Geometry check sheet. Reference: the model listing, model coordinates, mm. A direction names the side the tool comes from. Round coordinates to 2 decimals unless told otherwise and drop trailing zeros. Write each loop counter-clockwise with the first axis right and the second up, starting at its lowest first coordinate (ties: lowest second). Pieces come first, ordered by that corner, then holes. Notation, with made-up numbers: M 4,62.25 L 19,62.25 A19 cw 19,74.25 Z; hole C -7.5,22 d2. An arc over 180 degrees is marked long. Answer as CSV lines item,"result". Start each with the question number.
```python
from build123d import *

# Parameters (mm, degrees)
SKETCH1_W                  = 40
SKETCH1_H                  = 22
BOSS_EXTRUDE1_DEPTH        = 11
SKETCH2_W                  = 40
SKETCH2_H                  = 22
SKETCH2_R                  = 4
BOSS_EXTRUDE2_DEPTH        = 5
SKETCH3_W                  = 24.5
SKETCH3_H                  = 15.5
CUT_EXTRUDE1_DEPTH         = 7.75
FILLET1_R                  = 7.75
SKETCH4_R                  = 5
CUT_EXTRUDE2_DEPTH         = 36.805900352
SKETCH5_W                  = 8
SKETCH5_H                  = 8
SKETCH5_R                  = 1.905800151
BOSS_EXTRUDE3_DEPTH        = 6
CUT_EXTRUDE3_START         = -3
SKETCH6_R                  = 3
SKETCH6_R_2                = 1.905800151
CUT_EXTRUDE3_DEPTH         = 3
SKETCH7_W                  = 16
SKETCH7_H                  = 16.5
BOSS_EXTRUDE5_DEPTH        = 28
MIRROR14_COPY_1_SKETCH_W   = 8
MIRROR14_COPY_1_SKETCH_H   = 8
MIRROR14_COPY_1_SKETCH_R   = 1.905800151
MIRROR14_COPY_1_DEPTH      = 6
MIRROR14_START             = -3
MIRROR14_COPY_2_SKETCH_R   = 3
MIRROR14_COPY_2_SKETCH_R_2 = 1.905800151
MIRROR14_COPY_2_DEPTH      = 3
FILLET1_OF_MIRROR14_R      = 7.75
SKETCH9_W                  = 28
SKETCH9_H                  = 3
BOSS_EXTRUDE6_DEPTH        = 18
CUT_EXTRUDE4_DEPTH         = 10
CUT_EXTRUDE5_DEPTH         = 73.919476136
CUT_EXTRUDE5_DEPTH_BACK    = 73.919476136
SKETCH11_R                 = 1.75
CUT_EXTRUDE6_DEPTH         = 76.121568141
CUT_EXTRUDE6_DEPTH_BACK    = 76.121568141
SKETCH12_R                 = 1.75
FILLET2_R                  = 2
CUT_EXTRUDE12_START        = -3
SKETCH17_R                 = 1.75
CUT_EXTRUDE12_DEPTH        = 3
CUT_EXTRUDE13_DEPTH        = 74.097537578
CUT_EXTRUDE13_DEPTH_BACK   = 74.097537578
SKETCH18_W                 = 18
SKETCH18_H                 = 5
FILLET3_R                  = 2.5
CUT_EXTRUDE14_DEPTH        = 74.710582687
CUT_EXTRUDE15_START        = -10
SKETCH21_R                 = 1.75
CUT_EXTRUDE15_DEPTH        = 10
SKETCH20_W                 = 36.163748027
SKETCH20_H                 = 4
CUT_EXTRUDE16_DEPTH        = 13.5
SKETCH22_W                 = 6.75
SKETCH22_H                 = 13.5
CUT_EXTRUDE18_DEPTH        = 8


with BuildPart() as part:
    # Sketch1 → Boss-Extrude1 (new body)
    with BuildSketch(Plane(origin=(0, 0, 0), x_dir=(1, 0, 0), z_dir=(0, 1, 0))):
        Rectangle(SKETCH1_W, SKETCH1_H)
    boss_extrude1 = extrude(amount=BOSS_EXTRUDE1_DEPTH)

    # Sketch2 → Boss-Extrude2 (add)
    with BuildSketch(Plane(origin=(0, 0, 0), x_dir=(1, 0, 0), z_dir=(0, 1, 0))):
        Rectangle(SKETCH2_W, SKETCH2_H)
        with Locations(Location((0, 0, 0), (0, 0, 270))):
            Circle(SKETCH2_R, mode=Mode.SUBTRACT)
    boss_extrude2 = extrude(amount=-BOSS_EXTRUDE2_DEPTH)

    # Sketch3 → Cut-Extrude1 (cut)
    with BuildSketch(Plane(origin=(0, 11, 0), x_dir=(1, 0, 0), z_dir=(0, 1, 0))):
        Rectangle(SKETCH3_W, SKETCH3_H)
    cut_extrude1 = extrude(amount=-CUT_EXTRUDE1_DEPTH, mode=Mode.SUBTRACT)

    # Fillet1
    fillet1_edges = [part.edges().sort_by_distance(p)[0] for p in [
        (0, 3.25, 7.75),
        (0, 3.25, -7.75),
    ]]
    fillet(fillet1_edges, radius=FILLET1_R - 0.0001)  # a hair under: the kernel refuses the full size

    # Sketch4 → Cut-Extrude2 (cut, symmetric)
    with BuildSketch(Plane(origin=(-12.25, 0, 0), x_dir=(0, 0, -1), z_dir=(1, 0, 0))):
        with Locations((0, 11)):
            Circle(SKETCH4_R)
    cut_extrude2 = extrude(amount=CUT_EXTRUDE2_DEPTH, both=True, mode=Mode.SUBTRACT)

    # Sketch5 → Boss-Extrude3 (add)
    with BuildSketch(Plane(origin=(0, 11, 0), x_dir=(1, 0, 0), z_dir=(0, 1, 0))):
        with Locations((16, -15)):
            Rectangle(SKETCH5_W, SKETCH5_H)
        with Locations(Location((16, -15, 0), (0, 0, 270))):
            Circle(SKETCH5_R, mode=Mode.SUBTRACT)
    boss_extrude3 = extrude(amount=-BOSS_EXTRUDE3_DEPTH)

    # Sketch6 → Cut-Extrude3 (cut)
    with BuildSketch(Plane.XZ.offset(-5).offset(CUT_EXTRUDE3_START)):
        with Locations(Location((16, 15, 0), (0, 0, 270))):
            Circle(SKETCH6_R)
        with Locations(Location((16, 15, 0), (0, 0, 90))):
            Circle(SKETCH6_R_2, mode=Mode.SUBTRACT)
    cut_extrude3 = extrude(amount=CUT_EXTRUDE3_DEPTH, mode=Mode.SUBTRACT)

    # Mirror8: Boss-Extrude3, Cut-Extrude3 across plane
    add(boss_extrude3.mirror(Plane(origin=(0, 0, 0), x_dir=(0, 0, 1), z_dir=(1, 0, 0))))
    add(cut_extrude3.mirror(Plane(origin=(0, 0, 0), x_dir=(0, 0, 1), z_dir=(1, 0, 0))), mode=Mode.SUBTRACT)

    # Sketch7 → Boss-Extrude5 (add)
    with BuildSketch(Plane(origin=(0, 0, -11), x_dir=(-1, 0, 0), z_dir=(0, 0, -1))):
        with Locations((-12, 9.25)):
            Rectangle(SKETCH7_W, SKETCH7_H)
    extrude(amount=BOSS_EXTRUDE5_DEPTH)

    # Mirror14: Boss-Extrude1, Boss-Extrude2, Cut-Extrude1, Cut-Extrude2, Boss-Extrude3, Cut-Extrude3 across plane
    add(boss_extrude1.mirror(Plane.XY.offset(-25)))
    add(boss_extrude2.mirror(Plane.XY.offset(-25)))
    add(cut_extrude1.mirror(Plane.XY.offset(-25)), mode=Mode.SUBTRACT)
    add(cut_extrude2.mirror(Plane.XY.offset(-25)), mode=Mode.SUBTRACT)
    add(boss_extrude3.mirror(Plane.XY.offset(-25)))
    add(cut_extrude3.mirror(Plane.XY.offset(-25)), mode=Mode.SUBTRACT)

    # Mirror14 copy 1 sketch → Mirror14 copy 1 (add)
    with BuildSketch(Plane(origin=(0, 11, -50), x_dir=(-1, 0, 0), z_dir=(0, 1, 0))):
        with Locations((16, -15)):
            Rectangle(MIRROR14_COPY_1_SKETCH_W, MIRROR14_COPY_1_SKETCH_H)
        with Locations(Location((16, -15, 0), (0, 0, 270))):
            Circle(MIRROR14_COPY_1_SKETCH_R, mode=Mode.SUBTRACT)
    extrude(amount=-MIRROR14_COPY_1_DEPTH)

    # Mirror14 copy 2 sketch → Mirror14 copy 2 (cut)
    with BuildSketch(Plane(origin=(0, 5, -50), x_dir=(-1, 0, 0), z_dir=(0, -1, 0)).offset(MIRROR14_START)):
        with Locations(Location((16, 15, 0), (0, 0, 270))):
            Circle(MIRROR14_COPY_2_SKETCH_R)
        with Locations(Location((16, 15, 0), (0, 0, 90))):
            Circle(MIRROR14_COPY_2_SKETCH_R_2, mode=Mode.SUBTRACT)
    extrude(amount=MIRROR14_COPY_2_DEPTH, mode=Mode.SUBTRACT)

    # Fillet1 of Mirror14
    fillet1_of_mirror14_edges = [part.edges().sort_by_distance(p)[0] for p in [
        (0, 3.25, -57.75),
        (0, 3.25, -42.25),
    ]]
    fillet(fillet1_of_mirror14_edges, radius=FILLET1_OF_MIRROR14_R - 0.0001)  # a hair under: the kernel refuses the full size

    # Sketch9 → Boss-Extrude6 (add)
    with BuildSketch(Plane.ZY.offset(-4)):
        with Locations((-25, 2.5)):
            Rectangle(SKETCH9_W, SKETCH9_H)
    extrude(amount=BOSS_EXTRUDE6_DEPTH)

    # Sketch10 → Cut-Extrude4 (cut)
    with BuildSketch(Plane(origin=(0, 17.5, 0), x_dir=(1, 0, 0), z_dir=(0, 1, 0))):
        with BuildLine():
            Line((9, 26.25), (9, 23.75))
            Line((9, 23.75), (11.727178029, 23.75))
            ThreePointArc((11.727178029, 23.75), (11.931001031, 24.360286817), (12, 25))
            ThreePointArc((12, 25), (11.931001031, 25.639713183), (11.727178029, 26.25))
            Line((11.727178029, 26.25), (9, 26.25))
        make_face()
        with BuildLine():
            Line((11.727178029, 23.75), (9, 23.75))
            Line((9, 23.75), (9, 26.25))
            Line((9, 26.25), (11.727178029, 26.25))
            ThreePointArc((11.727178029, 26.25), (6, 25), (11.727178029, 23.75))
        make_face()
        with BuildLine():
            ThreePointArc((12, 25), (11.931001031, 24.360286817), (11.727178029, 23.75))
            Line((11.727178029, 23.75), (20, 23.75))
            Line((20, 23.75), (20, 26.25))
            Line((20, 26.25), (11.727178029, 26.25))
            ThreePointArc((11.727178029, 26.25), (11.931001031, 25.639713183), (12, 25))
        make_face()
    extrude(amount=-CUT_EXTRUDE4_DEPTH, mode=Mode.SUBTRACT)

    # Sketch11 → Cut-Extrude5 (cut, two sides: drawn at the far end of the back side and taken through both)
    with BuildSketch(Plane(origin=(0, 7.5, 0), x_dir=(1, 0, 0), z_dir=(0, 1, 0)).offset(-CUT_EXTRUDE5_DEPTH_BACK)):
        with Locations(Location((9, 25, 0), (0, 0, 270))):
            Circle(SKETCH11_R)
    extrude(amount=CUT_EXTRUDE5_DEPTH + CUT_EXTRUDE5_DEPTH_BACK, mode=Mode.SUBTRACT)

    # Sketch12 → Cut-Extrude6 (cut, two sides: drawn at the far end of the back side and taken through both)
    with BuildSketch(Plane.ZY.offset(-4).offset(-CUT_EXTRUDE6_DEPTH_BACK)):
        with Locations((-31, 11)):
            Circle(SKETCH12_R)
    extrude(amount=CUT_EXTRUDE6_DEPTH + CUT_EXTRUDE6_DEPTH_BACK, mode=Mode.SUBTRACT)

    # Fillet2
    fillet2_edges = [part.edges().sort_by_distance(p)[0] for p in [
        (11.727178029, 12.5, -23.75),
        (11.727178029, 12.5, -26.25),
    ]]
    fillet(fillet2_edges, radius=FILLET2_R)

    # Sketch17 → Cut-Extrude12 (cut)
    with BuildSketch(Plane.XZ.offset(-1).offset(CUT_EXTRUDE12_START)):
        Polygon((12.175426481, -25), (10.58771324, -22.25), (7.41228676, -22.25), (5.824573519, -25), (7.41228676, -27.75), (10.58771324, -27.75), align=None)
        with Locations(Location((9, -25, 0), (0, 0, 90))):
            Circle(SKETCH17_R, mode=Mode.SUBTRACT)
    extrude(amount=CUT_EXTRUDE12_DEPTH, mode=Mode.SUBTRACT)

    # Sketch18 → Cut-Extrude13 (cut, two sides: drawn at the far end of the back side and taken through both)
    with BuildSketch(Plane(origin=(0, 4, 0), x_dir=(1, 0, 0), z_dir=(0, 1, 0)).offset(-CUT_EXTRUDE13_DEPTH_BACK)):
        with Locations((-5, 25)):
            Rectangle(SKETCH18_W, SKETCH18_H)
    extrude(amount=CUT_EXTRUDE13_DEPTH + CUT_EXTRUDE13_DEPTH_BACK, mode=Mode.SUBTRACT)

    # Fillet3
    fillet3_edges = [part.edges().sort_by_distance(p)[0] for p in [
        (4, 2.5, -27.5),
        (4, 2.5, -22.5),
    ]]
    fillet(fillet3_edges, radius=FILLET3_R - 0.0001)  # a hair under: the kernel refuses the full size

    # Sketch19 → Cut-Extrude14 (cut, through all)
    with BuildSketch(Plane.XZ.offset(-1)):
        Polygon((20, -61), (20, -39), (-14, -39), (-20, -39), (-20, -61), align=None)
    extrude(amount=CUT_EXTRUDE14_DEPTH, mode=Mode.SUBTRACT)

    # Sketch21 → Cut-Extrude15 (cut)
    with BuildSketch(Plane(origin=(20, 0, 0), x_dir=(0, 0, -1), z_dir=(1, 0, 0)).offset(CUT_EXTRUDE15_START)):
        Polygon((31, 14.175426481), (28.25, 12.58771324), (28.25, 9.41228676), (31, 7.824573519), (33.75, 9.41228676), (33.75, 12.58771324), align=None)
        with Locations((31, 11)):
            Circle(SKETCH21_R, mode=Mode.SUBTRACT)
    extrude(amount=CUT_EXTRUDE15_DEPTH, mode=Mode.SUBTRACT)

    # Sketch20 → Cut-Extrude16 (cut)
    with BuildSketch(Plane(origin=(0, 17.5, 0), x_dir=(1, 0, 0), z_dir=(0, 1, 0))):
        with Locations((22.081874014, 37)):
            Rectangle(SKETCH20_W, SKETCH20_H)
    extrude(amount=-CUT_EXTRUDE16_DEPTH, mode=Mode.SUBTRACT)

    # Sketch22 → Cut-Extrude18 (cut)
    with BuildSketch(Plane(origin=(20, 0, 0), x_dir=(0, 0, -1), z_dir=(1, 0, 0))):
        with Locations((31.625, 10.75)):
            Rectangle(SKETCH22_W, SKETCH22_H)
    extrude(amount=-CUT_EXTRUDE18_DEPTH, mode=Mode.SUBTRACT)


solid = part.part
```
1) Section check B-B, the plane y = 15. Record the cut outline in (x, z), plus the area to 3 significant figures.
2) Access from +Z, -Z, +X, -X, +Y, -Y to the whole of each face (thin tool, end or side, straight path). Record for faces 1 (the flat face through (0, 11, 10)), 2 (the cylindrical face through (-3.905, -2.465, -0.867)), 3 (the flat face through (12.25, 5, -50)).
3) Mould release check, pull along Z, two halves, no side actions. Record for faces 4 (the flat face through (12.25, 5, 0)), 5 (the flat face through (16, 8, 19)), 6 (the flat face through (0, 11, -41)), 7 (the flat face through (0, 0, 0)): released by +Z, released by -Z, zero draft, split by the parting line, or undercut.
4) Section check C-C, the plane x = -16. Give the number of separate pieces and of enclosed holes in the cut face, plus the area to 3 significant figures.
5) Go/stop test with flat-tipped pins: pin 1 (13 mm diameter, centred on x = -2.5, y = 0.5, fed in from +Z); pin 2 (3 mm diameter, centred on x = 10, z = -25.5, fed in from -Y); pin 3 (13 mm diameter, centred on x = -3, y = 0.5, fed in from -Z). Record where each tip stops, or that it passes through.
6) Scan lines: line 1 (X direction, y = 6.8, z = 15); line 2 (Z direction, x = 9, y = 12.25); line 3 (Z direction, x = -4, y = 4.5). Record each from-to range of solid material in increasing order. Write a range as from..to.
Results:
1,outline,"M 4,-35 L 12,-35 L 12,-28.25 L 20,-28.25 L 20,-26.25 L 12.8,-26.25 A2 ccw 11.28,-26.95 A3 cw long 11.28,-23.05 A2 ccw 12.8,-23.75 L 20,-23.75 L 20,-11 L 4,-11 Z"
1,area,"281 mm^2"
2,face 1,"+Z, +X, -X, +Y"
2,face 2,"-Y"
2,face 3,"+Y"
3,face 4,"undercut"
3,face 5,"released by +Z"
3,face 6,"zero draft"
3,face 7,"undercut"
4,separate pieces,"4"
4,enclosed holes,"0"
4,area,"531 mm^2"
5,pin 1,"stops at z = 11"
5,pin 2,"stops at y = 4"
5,pin 3,"stops at z = -61"
6,line 1,"x = -20..-19, -13..-12, 12..13, 19..20"
6,line 2,"z = -35..-32.22, -29.78..-28, -22..-11"
6,line 3,"z = -61..-54.22, -45.78..-39, -11..-4.22, 4.22..11"
